Could you check a few things on this model? Use its own coordinates, in mm. Face numbers are marked on the shaded views. Give positions to 0.01 mm unless a question says otherwise; leave off trailing zeros. Write each loop counter-clockwise with the first axis right and the second up, starting at its lowest first coordinate (ties: lowest second). Pieces come first, ordered by that corner, then holes. Notation, with made-up numbers: (-1.75, 21.25) -> (9.25, 21.25) arc R15 cw to (9.25, 43.25) -> close; hole circle Ø8 at (-39, -14). An arc over 180 degrees is marked (long way). One line per question, with ' | ' between items.
from build123d import *

# Parameters (mm, degrees)
SKETCH1_W               = 204.5
SKETCH1_H               = 62.5
BOSS_EXTRUDE1_DEPTH     = 3
SKETCH2_R               = 8
BOSS_EXTRUDE2_DEPTH     = 7
SKETCH3_R               = 16
BOSS_EXTRUDE3_DEPTH     = 7
SKETCH4_R               = 2.165
CUT_EXTRUDE1_DEPTH      = 108.147678463
SKETCH5_R               = 2.165
CUT_EXTRUDE2_DEPTH      = 108.147678463
CUT_EXTRUDE3_DEPTH      = 7
MIRROR2_COPY_1_SKETCH_R = 2.165
MIRROR2_COPY_1_DEPTH    = 108.147678463
MIRROR2_COPY_2_DEPTH    = 7
MIRROR2_COPY_3_SKETCH_R = 2.165
MIRROR2_COPY_3_DEPTH    = 108.147678463
SKETCH7_R               = 12.5
CUT_EXTRUDE4_DEPTH      = 1.5
SKETCH9_R               = 11
CUT_EXTRUDE5_DEPTH      = 7
SKETCH10_R              = 8
CUT_EXTRUDE6_DEPTH      = 108.147678463
SKETCH11_R              = 4
CUT_EXTRUDE7_DEPTH      = 7


with BuildPart() as part:
    # Sketch1 → Boss-Extrude1 (new body)
    with BuildSketch(Plane.XY):
        Rectangle(SKETCH1_W, SKETCH1_H)
    extrude(amount=BOSS_EXTRUDE1_DEPTH)

    # Sketch2 → Boss-Extrude2 (add)
    with BuildSketch(Plane.XY.offset(3)):
        with Locations(Location((-87.5, 0, 0), (0, 0, 180))):
            Circle(SKETCH2_R)
        with Locations(Location((87.5, 0, 0), (0, 0, 180))):
            Circle(SKETCH2_R)
    extrude(amount=BOSS_EXTRUDE2_DEPTH)

    # Sketch3 → Boss-Extrude3 (add)
    with BuildSketch(Plane.XY.offset(3)):
        with Locations(Location((0, 0, 0), (0, 0, 180))):
            Circle(SKETCH3_R)
    extrude(amount=BOSS_EXTRUDE3_DEPTH)

    # Sketch4 → Cut-Extrude1 (cut, through all)
    with BuildSketch(Plane.XY.offset(3)):
        with Locations((-96.5, 9)):
            Circle(SKETCH4_R)
        with Locations((-96.5, -9)):
            Circle(SKETCH4_R)
    cut_extrude1 = extrude(amount=-CUT_EXTRUDE1_DEPTH, mode=Mode.SUBTRACT)

    # Sketch5 → Cut-Extrude2 (cut, through all)
    with BuildSketch(Plane.XY.offset(3)):
        with Locations((0, 26.875)):
            Circle(SKETCH5_R)
        with Locations((0, -26.875)):
            Circle(SKETCH5_R)
    extrude(amount=-CUT_EXTRUDE2_DEPTH, mode=Mode.SUBTRACT)

    # Sketch6 → Cut-Extrude3 (cut)
    with BuildSketch(Plane.XY.offset(3)):
        with BuildLine():
            Line((-102.25, 0), (-102.25, -9))
            ThreePointArc((-102.25, -9), (-101.935103767, -7.123261595), (-101.024905378, -5.452080705))
            Line((-101.024905378, -5.452080705), (-96.75, 0))
            Line((-96.75, 0), (-102.25, 0))
        make_face()
        with BuildLine():
            Line((-28, -8), (-82.092970466, -8))
            ThreePointArc((-82.092970466, -8), (-87.608403359, -9.22799932), (-92.081844276, -12.68))
            ThreePointArc((-92.081844276, -12.68), (-98.456796437, -14.406796437), (-102.25, -9))
            Line((-102.25, -9), (-102.25, -31.25))
            Line((-102.25, -31.25), (0, -31.25))
            ThreePointArc((0, -31.25), (-4.903490235, -29.873770102), (-9.063851408, -26.936148592))
            Line((-9.063851408, -26.936148592), (-28, -8))
        make_face()
    cut_extrude3 = extrude(amount=-CUT_EXTRUDE3_DEPTH, mode=Mode.SUBTRACT)

    # Mirror1: Cut-Extrude1, Cut-Extrude3 across plane
    add(cut_extrude1.mirror(Plane(origin=(0, 0, 0), x_dir=(0, 0, 1), z_dir=(1, 0, 0))), mode=Mode.SUBTRACT)
    add(cut_extrude3.mirror(Plane(origin=(0, 0, 0), x_dir=(0, 0, 1), z_dir=(1, 0, 0))), mode=Mode.SUBTRACT)

    # Mirror2: Cut-Extrude3 across plane
    add(cut_extrude3.mirror(Plane.ZX), mode=Mode.SUBTRACT)

    # Mirror2 copy 1 sketch → Mirror2 copy 1 (cut, through all)
    with BuildSketch(Plane(origin=(0, 0, 3), x_dir=(-1, 0, 0), z_dir=(0, 0, 1))):
        with Locations((-96.5, 9)):
            Circle(MIRROR2_COPY_1_SKETCH_R)
        with Locations((-96.5, -9)):
            Circle(MIRROR2_COPY_1_SKETCH_R)
    extrude(amount=-MIRROR2_COPY_1_DEPTH, mode=Mode.SUBTRACT)

    # Mirror2 copy 2 sketch → Mirror2 copy 2 (cut)
    with BuildSketch(Plane(origin=(0, 0, 3), x_dir=(-1, 0, 0), z_dir=(0, 0, 1))):
        with BuildLine():
            Line((-102.25, 0), (-102.25, -9))
            ThreePointArc((-102.25, -9), (-101.935103767, -7.123261595), (-101.024905378, -5.452080705))
            Line((-101.024905378, -5.452080705), (-96.75, 0))
            Line((-96.75, 0), (-102.25, 0))
        make_face()
        with BuildLine():
            Line((-28, -8), (-82.092970466, -8))
            ThreePointArc((-82.092970466, -8), (-87.608403359, -9.22799932), (-92.081844276, -12.68))
            ThreePointArc((-92.081844276, -12.68), (-98.456796437, -14.406796437), (-102.25, -9))
            Line((-102.25, -9), (-102.25, -31.25))
            Line((-102.25, -31.25), (0, -31.25))
            ThreePointArc((0, -31.25), (-4.903490235, -29.873770102), (-9.063851408, -26.936148592))
            Line((-9.063851408, -26.936148592), (-28, -8))
        make_face()
    extrude(amount=-MIRROR2_COPY_2_DEPTH, mode=Mode.SUBTRACT)

    # Mirror2 copy 3 sketch → Mirror2 copy 3 (cut, through all)
    with BuildSketch(Plane.XY.offset(3)):
        with Locations((-96.5, -9)):
            Circle(MIRROR2_COPY_3_SKETCH_R)
        with Locations((-96.5, 9)):
            Circle(MIRROR2_COPY_3_SKETCH_R)
    extrude(amount=-MIRROR2_COPY_3_DEPTH, mode=Mode.SUBTRACT)

    # Sketch7 → Cut-Extrude4 (cut)
    with BuildSketch(Plane.XY.offset(10)):
        Circle(SKETCH7_R)
    extrude(amount=-CUT_EXTRUDE4_DEPTH, mode=Mode.SUBTRACT)

    # Sketch9 → Cut-Extrude5 (cut)
    with BuildSketch(Plane.XY.offset(10)):
        Circle(SKETCH9_R)
    extrude(amount=-CUT_EXTRUDE5_DEPTH, mode=Mode.SUBTRACT)

    # Sketch10 → Cut-Extrude6 (cut, through all)
    with BuildSketch(Plane.XY.offset(3)):
        Circle(SKETCH10_R)
    extrude(amount=-CUT_EXTRUDE6_DEPTH, mode=Mode.SUBTRACT)

    # Sketch11 → Cut-Extrude7 (cut)
    with BuildSketch(Plane.XY.offset(10)):
        with Locations((-87.5, 0)):
            Circle(SKETCH11_R)
        with Locations((87.5, 0)):
            Circle(SKETCH11_R)
    extrude(amount=-CUT_EXTRUDE7_DEPTH, mode=Mode.SUBTRACT)


solid = part.part
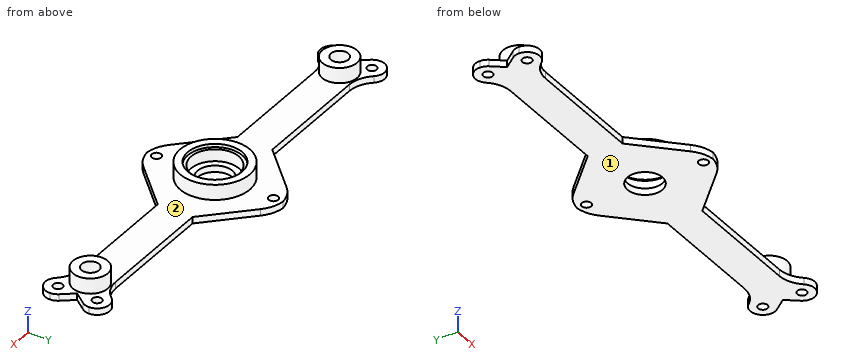
Q1. Imagine slicing it at A-A on z = 7. Please give me the cut outline in (x, y).
Answer below:
outline: circle Ø16 at (-87.5, 0); circle Ø32 at (0, 0); circle Ø16 at (87.5, 0); hole circle Ø8 at (-87.5, 0); hole circle Ø22 at (0, 0); hole circle Ø8 at (87.5, 0)
Q2. Imagine slicing it at C-C on y = -18. Please give me the cut outline in (x, z), and give its area (3 significant figures).
Answer below:
outline: (-18, 0) -> (18, 0) -> (18, 3) -> (-18, 3) -> close | area: 108 mm^2
Q3. If we mould it in two halves opening along X, with no side actions, what happens to the marked faces 1 and 2? For each: +X half, -X half, draft (parallel to the pull), parting line (faces both ways), or undercut.
Answer below:
face 1: draft | face 2: undercut
Q4. If I drill on line 1 along Y through (x, z) = (96.5, 0.75) (3 decimals); line 2 along Y through (x, z) = (0, 1.75); line 3 along Y through (x, z) = (0, 5.6), over which ranges is the centre line in solid material (lowest first)?
Answer below:
line 1: y = -14.75 to -11.165, -6.835 to 6.835, 11.165 to 14.75 | line 2: y = -31.25 to -29.04, -24.71 to -8, 8 to 24.71, 29.04 to 31.25 | line 3: y = -16 to -11, 11 to 16
Q5. Imagine slicing it at D-D on x = -87.5. Please give me the cut outline in (y, z), and give its area (3 significant figures).
Answer below:
outline: (-9.18, 0) -> (9.18, 0) -> (9.18, 3) -> (8, 3) -> (8, 10) -> (4, 10) -> (4, 3) -> (-4, 3) -> (-4, 10) -> (-8, 10) -> (-8, 3) -> (-9.18, 3) -> close | area: 111 mm^2
Q6. Will these pins go through, and if not, where does the flat tip stop? pin 1 (3.5 mm diameter, centred on x = -50, z = 1.5, fed in from +Y); pin 2 (1 mm diameter, centred on y = 12, z = 4.5, fed in from +X); pin 3 (4 mm diameter, centred on x = -87, y = 0.5, fed in from +Z).
Answer below:
pin 1: stops at y = 8 | pin 2: stops at x = 11.12 | pin 3: stops at z = 3
Q7. Imagine slicing it at B-B on x = 38.5. Please give me the cut outline in (y, z), and give its area (3 significant figures).
Answer below:
outline: (-8, 0) -> (8, 0) -> (8, 3) -> (-8, 3) -> close | area: 48.0 mm^2
